The listing builds one solid part. Answer for the finished solid, in the listing's coordinates (mm). Face numbers are marked on the shaded views. A direction names the side the tool comes from. Coordinates: 2 decimals unless noted, no trailing zeros. Order: outer loops, then holes, each group sorted by start corner. A loop starts at its lowest first (then second) coordinate and runs counter-clockwise, first axis right, second up. Notation, with made-up numbers: M 31,-34 L 50,-34 A24 ccw 50,-5 Z; hole C -34,46.5 d10. An arc over 180 degrees is marked long. One line per item, written item: value. Start each with the question number.
Q1. Straight lines are drawn through the part: line 1 along Z through (x, y) = (-32.5, 1.65); line 2 along X through (y, z) = (2.25, 21.5); line 3 along X through (y, z) = (1.5, 21). For each, find the intervals that lie inside material, in ascending order. Write a range as [from, to].
Q2. Determine the mould class of the marked faces 1, 2 and 3 for opening direction Z: pulls with the +Z half, pulls with the -Z half, needs draft (parallel to the pull), parting line crosses it, or undercut.
Q3. Each of these flat-tipped pins is pushed along its axis until it touches: pin 1 Ø6 at (x, y) = (42.5, 7) entering from -Z; pin 2 Ø5.5 at (x, z) = (32.5, -21.5) entering from +Y; pin 3 Ø2 at (x, y) = (41, 21) entering from +Z; pin 4 Ø3 at (x, z) = (-32.5, 21.5) entering from +Y. Where does it stop, or does it pass through?
Q4. The part is cut by section A-A on x = -32.5. Give the vertices of the cut face in (y, z).
Q5. The part is cut by section D-D on y = 11.5. Give the vertices of the cut face in (x, z).
Q6. For the marked faces 4, 5 and 6, determine the directions among +Z, -Z, +X, -X, +Y, -Y from which every point of the face is accessible in a straight line to the end or side of a thin tool.
Q7. The part is cut by section B-B on z = 5. Give the vertices of the cut face in (x, y).
Q8. The part is cut by section C-C on z = -21.5. Give the vertices of the cut face in (x, y).
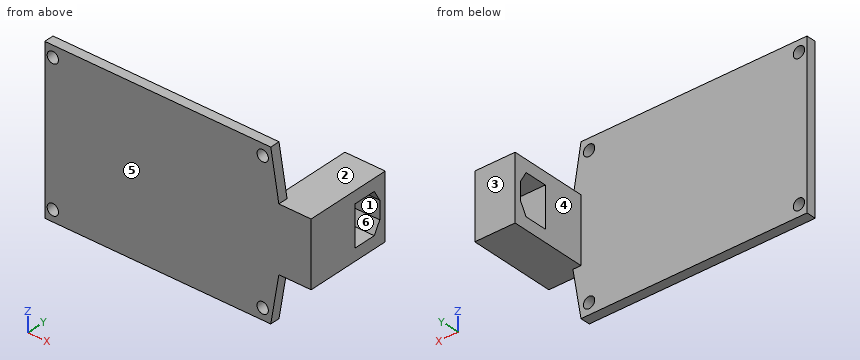
```python
from build123d import *

# Parameters (mm, degrees)
SKETCH1_W                                  = 70
SKETCH1_H                                  = 50
BOSS_EXTRUDE1_DEPTH                        = 3
SKETCH2_R                                  = 1.75
CUT_EXTRUDE1_DEPTH                         = 10
MIRROR1_AT_THE_SECOND_PLANE_COPY_1_SKETC_R = 1.75
MIRROR1_AT_THE_SECOND_PLANE_COPY_1_DEPTH   = 10
SKETCH4_W                                  = 2.5
SKETCH4_H                                  = 10
BOSS_EXTRUDE2_DEPTH                        = 28
BOSS_EXTRUDE3_DEPTH                        = 3
CUT_EXTRUDE2_DEPTH                         = 3
BOSS_EXTRUDE4_DEPTH                        = 10
BOSS_EXTRUDE5_DEPTH                        = 10
SKETCH11_W                                 = 20
SKETCH11_H                                 = 1
CUT_EXTRUDE3_DEPTH                         = 10


with BuildPart() as part:
    # Sketch1 → Boss-Extrude1 (new body)
    with BuildSketch(Plane(origin=(0, 0, 0), x_dir=(1, 0, 0), z_dir=(0, 1, 0))):
        Rectangle(SKETCH1_W, SKETCH1_H)
    extrude(amount=BOSS_EXTRUDE1_DEPTH)

    # Sketch2 → Cut-Extrude1 (cut)
    with BuildSketch(Plane(origin=(0, 3, 0), x_dir=(1, 0, 0), z_dir=(0, 1, 0))):
        with Locations(Location((32.5, -21.5, 0), (0, 0, 270))):
            Circle(SKETCH2_R)
    cut_extrude1 = extrude(amount=-CUT_EXTRUDE1_DEPTH, mode=Mode.SUBTRACT)

    # Mirror1: Cut-Extrude1 across plane
    add(cut_extrude1.mirror(Plane.XY), mode=Mode.SUBTRACT)

    # Mirror1 at the second plane: Cut-Extrude1 across plane
    add(cut_extrude1.mirror(Plane(origin=(0, 0, 0), x_dir=(0, 0, 1), z_dir=(1, 0, 0))), mode=Mode.SUBTRACT)

    # Mirror1 at the second plane copy 1 sketc → Mirror1 at the second plane copy 1 (cut)
    with BuildSketch(Plane(origin=(0, 3, 0), x_dir=(-1, 0, 0), z_dir=(0, 1, 0))):
        with Locations(Location((32.5, -21.5, 0), (0, 0, 270))):
            Circle(MIRROR1_AT_THE_SECOND_PLANE_COPY_1_SKETC_R)
    extrude(amount=-MIRROR1_AT_THE_SECOND_PLANE_COPY_1_DEPTH, mode=Mode.SUBTRACT)

    # Sketch4 → Boss-Extrude2 (add)
    with BuildSketch(Plane(origin=(0, 0, 0), x_dir=(1, 0, 0), z_dir=(0, 1, 0))):
        with Locations((36.25, -5)):
            Rectangle(SKETCH4_W, SKETCH4_H)
        with Locations((36.25, 5)):
            Rectangle(SKETCH4_W, SKETCH4_H)
    extrude(amount=BOSS_EXTRUDE2_DEPTH)

    # Sketch7 → Boss-Extrude3 (add)
    with BuildSketch(Plane(origin=(0, 3, 0), x_dir=(1, 0, 0), z_dir=(0, 1, 0))):
        Polygon((35, -10), (35, -25), (37.5, -10), align=None)
    boss_extrude3 = extrude(amount=-BOSS_EXTRUDE3_DEPTH)

    # Mirror2: Boss-Extrude3 across plane
    add(boss_extrude3.mirror(Plane.XY))

    # Sketch8 → Cut-Extrude2 (cut)
    with BuildSketch(Plane(origin=(37.5, 0, 0), x_dir=(0, 0, -1), z_dir=(1, 0, 0))):
        Polygon((-2.785898385, 25), (-6.25, 23), (-6.25, 16), (6.25, 16), (6.25, 23), (2.785898385, 25), align=None)
    extrude(amount=-CUT_EXTRUDE2_DEPTH, mode=Mode.SUBTRACT)

    # Sketch9 → Boss-Extrude4 (add)
    with BuildSketch(Plane(origin=(37.5, 0, 0), x_dir=(0, 0, -1), z_dir=(1, 0, 0))):
        Polygon((-6.75, 15.5), (6.75, 15.5), (6.75, 23.288675135), (2.919872981, 25.5), (-2.919872981, 25.5), (-6.75, 23.288675135), align=None)
        Polygon((-6.25, 23), (-6.25, 16), (6.25, 16), (6.25, 23), (2.785898385, 25), (-2.785898385, 25), align=None, mode=Mode.SUBTRACT)
    extrude(amount=BOSS_EXTRUDE4_DEPTH)

    # Sketch10 → Boss-Extrude5 (add)
    with BuildSketch(Plane(origin=(37.5, 0, 0), x_dir=(0, 0, -1), z_dir=(1, 0, 0))):
        Polygon((10, 27), (-10, 27), (-10, 3), (-10, 0), (10, 0), (10, 3), align=None)
        Polygon((-6.75, 15.5), (-6.75, 23.288675135), (-2.919872981, 25.5), (2.919872981, 25.5), (6.75, 23.288675135), (6.75, 15.5), align=None, mode=Mode.SUBTRACT)
    extrude(amount=BOSS_EXTRUDE5_DEPTH)

    # Sketch11 → Cut-Extrude3 (cut)
    with BuildSketch(Plane(origin=(37.5, 0, 0), x_dir=(0, 0, -1), z_dir=(1, 0, 0))):
        with Locations((0, 27.5)):
            Rectangle(SKETCH11_W, SKETCH11_H)
    extrude(amount=-CUT_EXTRUDE3_DEPTH, mode=Mode.SUBTRACT)


solid = part.part
```
Output:
1. line 1: z = [-25, -23.25], [-19.75, 19.75], [23.25, 25]
1. line 2: x = [-35, -34.25], [-30.75, 30.75], [34.25, 35.58]
1. line 3: x = [-35, -34.18], [-30.82, 30.82], [34.18, 35.67]
2. face 1: undercut
2. face 2: pulls with the +Z half
2. face 3: needs draft
3. pin 1: stops at z = -10
3. pin 2: stops at y = 3
3. pin 3: stops at z = 10
3. pin 4: passes through
4. outline: M 0,-25 L 3,-25 L 3,-23.25 L 0,-23.25 Z; M 0,-19.75 L 3,-19.75 L 3,19.75 L 0,19.75 Z; M 0,23.25 L 3,23.25 L 3,25 L 0,25 Z
5. outline: M 35,-10 L 47.5,-10 L 47.5,10 L 35,10 Z
6. face 4: +Z, -Z, -X, +Y
6. face 5: +Z, -Z, +X, -X, -Y
6. face 6: +X, -X
7. outline: M -35,0 L 47.5,0 L 47.5,16 L 35,16 L 35,3 L -35,3 Z; M 35,23.72 L 47.5,23.72 L 47.5,27 L 35,27 Z
8. outline: M -35,0 L -34.25,0 L -34.25,3 L -35,3 Z; M -30.75,0 L 30.75,0 L 30.75,3 L -30.75,3 Z; M 34.25,0 L 35.58,0 L 35.58,3 L 34.25,3 Z
